Can you work these out from the drawing? Everything is in mm from the part's minimum corner. Give positions to 0.01 mm unless a question says otherwise; leave off trailing zeros. Loops run counter-clockwise (first coordinate to the right, second up) from the corner with the lowest first, then second, coordinate; pieces in that order, holes last. Notation, with made-up numbers: (46, 3) - (50, 3) arc R21 ccw to (50, 22) - close; hole circle Ø3 at (-12.5, -35). An arc over 180 degrees is marked (long way). One line per item, written item: value. Start each with the question number.
Q1. I want a section at C-C (z = 9.5). Please give me the cut outline in (x, y).
Q2. I'm going to push flat-ended pins straight in: P1, Ø1.5, axis at x = 14.5, z = 43.5, coming from the +Y side; P2, Ø2, axis at y = 7.5, z = 4, coming from the -X side; P3, Ø1.8, axis at x = 16, y = 3, coming from the -Z side. Where does each tip first touch, or does it pass through?
Q3. If I drill on line 1 (Z direction, x = 4.5, y = 0.3); line 2 (X direction, y = 0.55, z = 30.25); line 3 (Y direction, x = 14, z = 35.5), over which ranges is the centre line in solid material (lowest first)? Write a range as from..to.
Q4. I want a section at B-B (x = 19.5). Please give me the cut outline in (y, z).
Q5. I want a section at A-A (z = 24.5). Please give me the cut outline in (x, y).
Q6. I want a section at D-D (y = 8.25). Please give me the cut outline in (x, z), then the cut area to 3 significant figures.
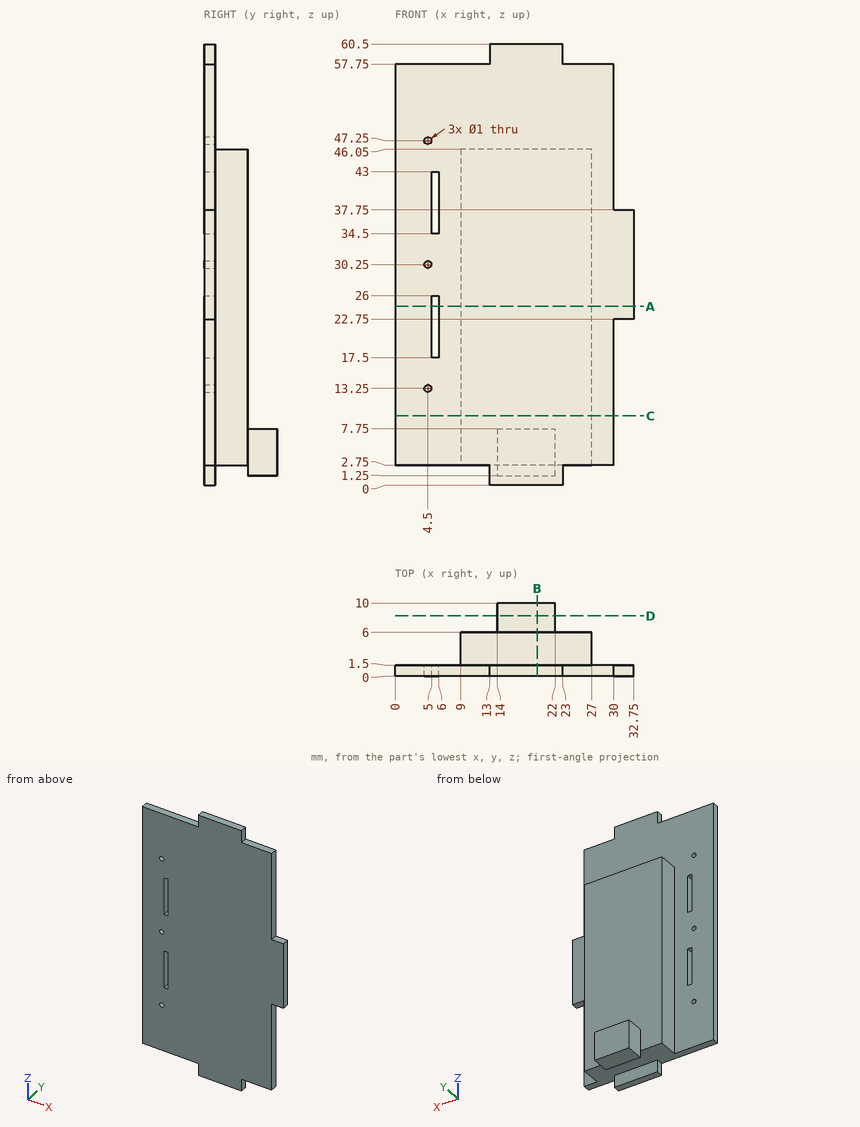
Worked answers:
1. outline: (0, 0) - (30, 0) - (30, 1.5) - (27, 1.5) - (27, 6) - (9, 6) - (9, 1.5) - (0, 1.5) - close
2. P1: stops at y = 6
2. P2: stops at x = 14
2. P3: stops at z = 2.75
3. line 1: z = 2.75..12.75, 13.75..29.75, 30.75..46.75, 47.75..57.75
3. line 2: x = 0..4, 5..32.75
3. line 3: y = 0..6
4. outline: (0, 0) - (1.5, 0) - (1.5, 2.75) - (6, 2.75) - (6, 1.25) - (10, 1.25) - (10, 7.75) - (6, 7.75) - (6, 46.05) - (1.5, 46.05) - (1.5, 60.5) - (0, 60.5) - close
5. outline: (0, 0) - (5, 0) - (5, 1.5) - (0, 1.5) - close; (6, 0) - (32.75, 0) - (32.75, 1.5) - (27, 1.5) - (27, 6) - (9, 6) - (9, 1.5) - (6, 1.5) - close
6. outline: (14, 1.25) - (22, 1.25) - (22, 7.75) - (14, 7.75) - close
6. area: 52.0 mm²
